Could you check a few things on this model? Use its own coordinates, in mm. Face numbers are marked on the shaded views. Give positions to 0.01 mm unless a question says otherwise; leave off trailing zeros. Order: outer loops, then holes, each group sorted by start corner. A loop starts at its lowest first (then second) coordinate and runs counter-clockwise, first axis right, second up.
(1) Imagine slicing it at B-B, the plane y = 0. State how many separate pieces and enclosed holes the cut face has, then the cut area to 3 significant figures.
(2) Imagine slicing it at C-C, the plane z = 0.15. Write out the boundary of the cut face in (x, y) (1 decimal), then the cut area to 3 significant figures.
(3) If I drill on probe 1 along X at (y, z) = (-3.25, 0.5); probe 2 along Y at (x, z) = (0, 1.05); probe 3 along Y at (x, z) = (0.75, 0.8), over which ranges is the centre line in solid material (lowest first)?
(4) Will these pins go through, and if not, where does the flat tip stop? pin 1 (1 mm diameter, centred on x = -2, z = -0.5, fed in from +Y); pin 2 (1 mm diameter, centred on x = -3, y = -4.5, fed in from +Z).
(5) If we mould it in two halves opening along X, with no side actions, what happens to the marked faces 1, 2 and 3? For each: released by +X, released by -X, zero draft, split by the parting line, or undercut.
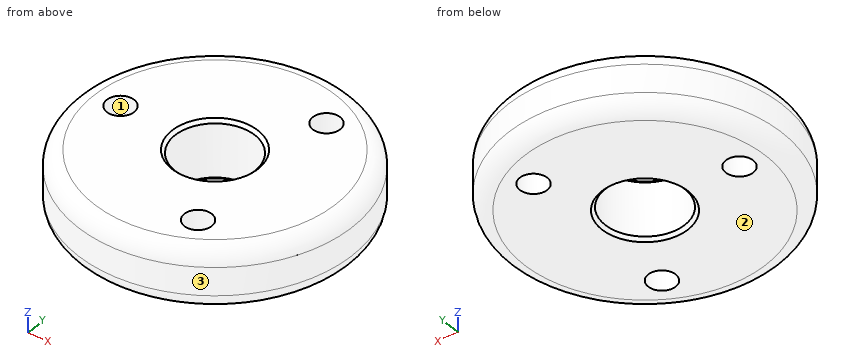
Autodesk Inventor part; units mm, degrees
ref_plane "YZ Plane" through (0, 0, 0) normal (1, 0, 0) x (0, 1, 0)
ref_plane "XZ Plane" through (0, 0, 0) normal (0, 1, 0) x (-1, 0, 0)
ref_plane "XY Plane" through (0, 0, 0) normal (0, 0, 1) x (1, 0, 0)
sketch "Sketch1" plane through (0, 0, 0) normal (0, 0, 1) x (1, 0, 0)
  circle A0 centre (0, 0) radius 1.5875
  circle A1 centre (0, 0) radius 5.461
  dimension "d0" = 3.175
  dimension "d1" = 10.922
extrude "Extrusion1" add sketch "Sketch1" along normal mid plane 2.3813
fillet "Fillet1" radius 0.635 2 edges at (-5.461, 0, 1.1906) (-5.461, 0, -1.1906)
chamfer "Chamfer1" distance 0.127 angle 45 2 edges at (-1.5875, 0, 1.1906) (-1.5875, 0, -1.1906)
sketch "Sketch2" plane through (0, 0, 1.1906) normal (0, 0, 1) x (1, 0, 0)
  circle A0 centre (-3.81, 0) radius 0.5461
  point P0 (0, 0)
  dimension "d8" = 1.0922
  dimension "d9" = 3.81
extrude "Extrusion2" cut sketch "Sketch2" along normal through all both and the other way through all
pattern_circular "Circular Pattern1" count 3 over 360 about axis through (0, 0, -10) along (0, 0, 1) of "Extrusion2"
properties part number "Piston of Suspension"
Answer block:
1. separate pieces: 3
1. enclosed holes: 0
1. area: 15.5 mm2
2. outline: circle Ø10.9 at (0, 0); hole circle Ø1.1 at (-3.8, 0); hole circle Ø3.2 at (0, 0); hole circle Ø1.1 at (1.9, -3.3); hole circle Ø1.1 at (1.9, 3.3)
2. area: 83.0 mm2
3. probe 1: x = -4.39 to 1.36, 2.45 to 4.39
3. probe 2: y = -5.22 to -1.59, 1.59 to 5.22
3. probe 3: y = -5.36 to -1.4, 1.4 to 5.36
4. pin 1: stops at y = 5.25
4. pin 2: stops at z = 1.19
5. face 1: undercut
5. face 2: zero draft
5. face 3: split by the parting line
